from build123d import *

# Parameters (mm, degrees)
F1_DEPTH  = 171.196
F3_W      = 47.717366
F3_H      = 50.21789
F4_DEPTH  = 198.12
F5_R      = 2.706537
F6_DEPTH  = 205.232
F7_R      = 1.888805
F8_DEPTH  = 241.046
F9_R      = 2.795925
F10_DEPTH = 243.84
F11_R     = 3.182079
F12_DEPTH = 208.534
F13_R     = 2.616602
F14_DEPTH = 201.422
F15_R     = 2.301935
F16_DEPTH = 190.754
F17_W     = 47.983054
F17_H     = 58.105506
F18_DEPTH = 171.196
F19_W     = 48.245978
F19_H     = 57.579667
F20_DEPTH = 182.626


with BuildPart() as f1:
    # F0 (on Front) → F1 (new body)
    with BuildSketch(Plane.XZ):
        with BuildLine():
            ThreePointArc((49.965762, 0), (25.475067, 7.042813), (0, 6.397561))
            ThreePointArc((0, 6.397561), (-3.740285, 3.19878), (0, 0))
            Line((0, 0), (49.965762, 0))
        make_face()
    extrude(amount=F1_DEPTH)

    # F3 (on offset) → F4 (cut)
    with BuildSketch(Plane.XY.offset(-75.692)):
        with Locations((23.858683, -145.044405)):
            Rectangle(F3_W, F3_H)
    extrude(amount=F4_DEPTH, mode=Mode.SUBTRACT)

    # F5 (on Front) → F6 (cut)
    with BuildSketch(Plane.XZ):
        with Locations((0, 3.158289)):
            Circle(F5_R)
    extrude(amount=F6_DEPTH, mode=Mode.SUBTRACT)

    # F7 (on Front) → F8 (cut)
    with BuildSketch(Plane.XZ):
        with Locations((34.417257, 2.834362)):
            Circle(F7_R)
    extrude(amount=F8_DEPTH, mode=Mode.SUBTRACT)

    # F9 (on Front) → F10 (cut)
    with BuildSketch(Plane.XZ):
        with Locations((7.531306, 3.806144)):
            Circle(F9_R)
    extrude(amount=F10_DEPTH, mode=Mode.SUBTRACT)

    # F11 (on Front) → F12 (cut)
    with BuildSketch(Plane.XZ):
        with Locations((14.333775, 3.806144)):
            Circle(F11_R)
    extrude(amount=F12_DEPTH, mode=Mode.SUBTRACT)

    # F13 (on Front) → F14 (cut)
    with BuildSketch(Plane.XZ):
        with Locations((21.136245, 3.482217)):
            Circle(F13_R)
    extrude(amount=F14_DEPTH, mode=Mode.SUBTRACT)

    # F15 (on Front) → F16 (cut)
    with BuildSketch(Plane.XZ):
        with Locations((27.776752, 3.64418)):
            Circle(F15_R)
    extrude(amount=F16_DEPTH, mode=Mode.SUBTRACT)

    # F17 (on offset) → F18 (cut)
    with BuildSketch(Plane.XY.offset(-75.692)):
        with Locations((23.991527, -89.565333)):
            Rectangle(F17_W, F17_H)
    extrude(amount=F18_DEPTH, mode=Mode.SUBTRACT)

    # F19 (on offset) → F20 (cut)
    with BuildSketch(Plane.XY.offset(-75.692)):
        with Locations((24.122989, -30.671063)):
            Rectangle(F19_W, F19_H)
    extrude(amount=F20_DEPTH, mode=Mode.SUBTRACT)


solid = f1.part
Design review of the part built by this model. Coordinates are the model's own, in mm. Round coordinates to 2 decimals unless told otherwise and drop trailing zeros. Use a Markdown table: item, result. Add a question column.
1. Clearance check with flat-ended pins moving along their axes: pin 1 (1.5 mm diameter, centred on x = 38, z = 6, fed in from -Y); pin 2 (1.5 mm diameter, centred on y = -33.5, z = 5, fed in from -X); pin 3 (1.1 mm diameter, centred on y = -138.5, z = 0.5, fed in from -X). State where each tip first meets the part, or that it passes through.
2. Wall thickness on probe 1 along Y at (x, z) = (19, 7.25); probe 2 along Z at (x, y) = (-1, -156); probe 3 along X at (y, z) = (-116, 4.5): over which ranges is each line inside the solid? List them lowest first.
3. We need section B-B (x = 22). Count the separate pieces of the cut face and the enclosed holes in it, then the cut area to 3 significant figures.
4. Mouldability with a two-part tool opening along Z and no side actions: class faces 1 (the face through (49, -73, 0)), 2 (the face through (-2.704, -84.4, 3.277)), 3 (the face through (24, -170.153, 2)) as +Z half, -Z half, draft (parallel to the pull), parting line (faces both ways), or undercut.
Output:
| question | item | result |
|---|---|---|
| 1 | pin 1 | passes through |
| 1 | pin 2 | stops at x = -3.56 |
| 1 | pin 3 | stops at x = -2.92 |
| 2 | probe 1 | y = -171.2 to -170.15, -119.94 to -118.62, -60.51 to -59.46, -1.88 to 0 |
| 2 | probe 2 | z = 0 to 0.64, 5.67 to 6.4 |
| 2 | probe 3 | x = -3.47 to -2.35 |
| 3 | separate pieces | 8 |
| 3 | enclosed holes | 0 |
| 3 | area | 13.1 mm2 |
| 4 | face 1 | -Z half |
| 4 | face 2 | undercut |
| 4 | face 3 | draft |
